For this review, take the finished solid that the model builds, in its own axes (mm). Face numbers are marked on the shaded views. A direction names the side the tool comes from. Round coordinates to 2 decimals unless told otherwise and drop trailing zeros. Loops run counter-clockwise (first coordinate to the right, second up) from the corner with the lowest first, then second, coordinate; pieces in that order, holes last.
1. Draft analysis for pull direction Y (two halves, no side actions). For the marked faces 4, 5, 6 and 7, state which applies: released by +Y, released by -Y, zero draft, split by the parting line, or undercut.
2. Clearance check with flat-ended pins moving along their axes: pin 1 Ø4 at (x, z) = (-2, 6.5) entering from +Y; pin 2 Ø2.5 at (x, z) = (-3, 8.5) entering from -Y; pin 3 Ø3.5 at (x, y) = (12, 15.25) entering from -Z; pin 4 Ø2 at (x, y) = (51, 43) entering from +Z. State where each tip first meets the part, or that it passes through.
3. Tool access review of the marked faces 1, 2 and 3: name each direction out of +Z, -Z, +X, -X, +Y, -Y from which nothing blocks a thin tool from reaching the whole face with its end or side.
4. Consider section B-B on x = -11.5. State the section outline as (y, z) points.
5. To check wall thickness, follow line 1 along Y through (x, z) = (5, 0.4); line 2 along Y through (x, z) = (17, 10.75); line 3 along Z through (x, y) = (7, 15). State the ranges of each line that lie inside material, in increasing order.
from build123d import *

# Parameters (mm, degrees)
F0_W     = 84.554
F0_H     = 110
F0_R     = 3
F0_R_2   = 1.778
F1_DEPTH = 2
F2_DEPTH = 12
F3_DEPTH = 12
F4_R     = 4.99999
F5_R     = 5
F6_R     = 1
F7_DEPTH = 25
F8_DEPTH = 25


# Not quite as in the source:
# - a fillet or chamfer is up to 0.001 mm smaller than in the source, because OpenCascade refuses the exact size
# - a feature names something its author has since deleted; it is built from what else it names


with BuildPart() as f1:
    # F0 (on Top) → F1 (new body)
    with BuildSketch(Plane.XY):
        with Locations((17.277, 35)):
            Rectangle(F0_W, F0_H)
        with Locations((12, 15.25)):
            Circle(F0_R, mode=Mode.SUBTRACT)
        Polygon((0, 5), (0, 0), (34.554, 0), (34.554, 5), (39.554, 5), (39.554, -10), (-5, -10), (-5, 5), align=None, mode=Mode.SUBTRACT)
        with Locations((17.277, 4.95)):
            Circle(F0_R_2, mode=Mode.SUBTRACT)
        with Locations((22.554, 25.25)):
            Circle(F0_R, mode=Mode.SUBTRACT)
        with Locations((12, 35.25)):
            Circle(F0_R, mode=Mode.SUBTRACT)
        with Locations((12, 55.25)):
            Circle(F0_R, mode=Mode.SUBTRACT)
        with Locations((22.554, 45.25)):
            Circle(F0_R, mode=Mode.SUBTRACT)
        with Locations((17.277, 65.05)):
            Circle(F0_R_2, mode=Mode.SUBTRACT)
        Polygon((6.482, 70), (0, 56.776), (0, 51.776), (-5, 51.776), (-5, 80), (39.554, 80), (39.554, 51.776), (34.554, 51.776), (34.554, 56.776), (28.072, 70), align=None, mode=Mode.SUBTRACT)
    extrude(amount=F1_DEPTH)

    # F0 (on Top) → F2 (join)
    with BuildSketch(Plane.XY):
        Polygon((0, 51.776), (0, 56.776), (6.482, 70), (28.072, 70), (34.554, 56.776), (34.554, 51.776), (39.554, 51.776), (39.554, 80), (-5, 80), (-5, 51.776), align=None)
    extrude(amount=F2_DEPTH)

    # F0 (on Top) → F3 (join)
    with BuildSketch(Plane.XY):
        Polygon((34.554, 0), (0, 0), (0, 5), (-5, 5), (-5, -10), (39.554, -10), (39.554, 5), (34.554, 5), align=None)
    extrude(amount=F3_DEPTH)

    # F4 (radius 5 in the source; OpenCascade refuses exactly that, so slightly less here)
    f4_edges = [f1.edges().sort_by_distance(p)[0] for p in [
        (6.482, 70, 7),
        (28.072, 70, 7),
        (0, 56.776, 7),
        (34.554, 56.776, 7),
        (34.554, 0, 7),
        (0, 0, 7),
        (59.554, -20, 1),
        (59.554, 90, 1),
        (-25, 90, 1),
        (-25, -20, 1),
    ]]
    fillet(f4_edges, radius=F4_R)

    # F5
    f5_edges = [f1.edges().sort_by_distance(p)[0] for p in [
        (-5, -10, 7),
        (39.554, -10, 7),
        (39.554, 80, 7),
        (-5, 80, 7),
    ]]
    fillet(f5_edges, radius=F5_R)

    # F6 (on face) → F7 (cut)
    with BuildSketch(Plane.XY.offset(2)):
        with Locations((5, 55.25)):
            Circle(F6_R)
        with Locations((19, 55.25)):
            Circle(F6_R)
        with Locations((19, 35.25)):
            Circle(F6_R)
        with Locations((5, 35.25)):
            Circle(F6_R)
        with Locations((15.554, 25.25)):
            Circle(F6_R)
        with Locations((29.554, 25.25)):
            Circle(F6_R)
    extrude(amount=-F7_DEPTH, mode=Mode.SUBTRACT)

    # F6 (on face) → F8 (cut)
    with BuildSketch(Plane.XY.offset(2)):
        with Locations((5, 55.25)):
            Circle(F6_R)
        with Locations((19, 55.25)):
            Circle(F6_R)
        with Locations((19, 35.25)):
            Circle(F6_R)
        with Locations((5, 35.25)):
            Circle(F6_R)
        with Locations((15.554, 25.25)):
            Circle(F6_R)
        with Locations((29.554, 25.25)):
            Circle(F6_R)
        with Locations((15.554, 45.25)):
            Circle(F6_R)
        with Locations((29.554, 45.25)):
            Circle(F6_R)
        with Locations((5, 15.25)):
            Circle(F6_R)
        with Locations((19, 15.25)):
            Circle(F6_R)
    extrude(amount=-F8_DEPTH, mode=Mode.SUBTRACT)


solid = f1.part
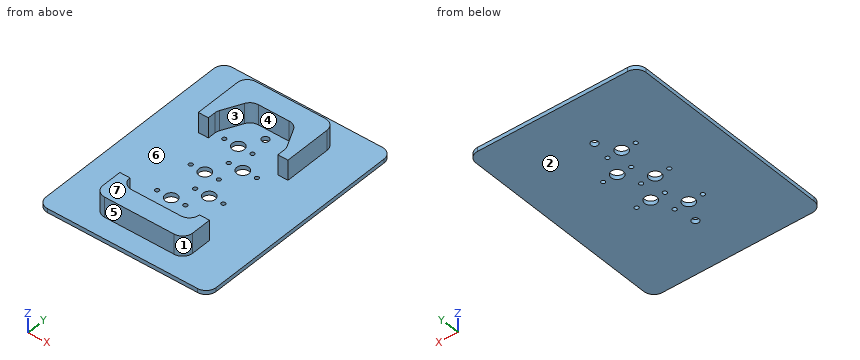
Resolved:
1. face 4: undercut
1. face 5: released by -Y
1. face 6: undercut
1. face 7: zero draft
2. pin 1: stops at y = 80
2. pin 2: stops at y = -9.68
2. pin 3: passes through
2. pin 4: stops at z = 2
3. face 1: +Z, +X, -Y
3. face 2: -Z, +X, -X, +Y, -Y
3. face 3: +Z
4. outline: (-20, 0) - (90, 0) - (90, 2) - (-20, 2) - close
5. line 1: y = -20 to 14.25, 16.25 to 34.25, 36.25 to 54.25, 56.25 to 90
5. line 2: y = -10 to 0, 70 to 80
5. line 3: z = 0 to 2
